CAD build for the part. Positions are in the model's coordinates, mm. A direction names the side the tool comes from. Give positions to 0.01 mm unless a question says otherwise; leave off trailing zeros. Loops run counter-clockwise (first coordinate to the right, second up) from the corner with the lowest first, then second, coordinate; pieces in that order, holes last.
```python
from build123d import *

# Parameters (mm, degrees)
F1_DEPTH = 6
F3_DEPTH = 2
F4_R     = 2.25
F5_DEPTH = 8.001
F6_R     = 3.75
F7_DEPTH = 2
F8_SIZE  = 3


with BuildPart() as f1:
    # F0 (on Top) → F1 (new body)
    with BuildSketch(Plane.XY):
        Polygon((0, 40), (0, 0), (60, 0), (60, 20), (20, 40), align=None)
    extrude(amount=F1_DEPTH)

    # F2 (on face) → F3 (join)
    with BuildSketch(Plane.XY.offset(6)):
        Polygon((12.71, 40), (7.29, 40), (7.29, 0), (10, 0), (12.71, 0), align=None)
        Polygon((60, 7.29), (60, 12.71), (20, 12.71), (20, 10), (20, 7.29), align=None)
    extrude(amount=F3_DEPTH)

    # F4 (on face) → F5 (cut, through all)
    with BuildSketch(Plane(origin=(0, 0, 0), x_dir=(1, 0, 0), z_dir=(0, 0, -1))):
        with Locations((10, -10)):
            Circle(F4_R)
        with Locations((50, -10)):
            Circle(F4_R)
        with Locations((10, -30)):
            Circle(F4_R)
        with Locations((30, -10)):
            Circle(F4_R)
    extrude(amount=-F5_DEPTH, mode=Mode.SUBTRACT)

    # F6 (on face) → F7 (cut)
    with BuildSketch(Plane(origin=(0, 0, 0), x_dir=(1, 0, 0), z_dir=(0, 0, -1))):
        with Locations((10, -10)):
            Circle(F6_R)
        with Locations((30, -10)):
            Circle(F6_R)
        with Locations((50, -10)):
            Circle(F6_R)
        with Locations((10, -30)):
            Circle(F6_R)
    extrude(amount=-F7_DEPTH, mode=Mode.SUBTRACT)

    # F8
    f8_edges = [f1.edges().sort_by_distance(p)[0] for p in [
        (30, 0, 0),
        (0, 20, 0),
        (60, 10, 0),
        (10, 40, 0),
        (40, 30, 0),
    ]]
    chamfer(f8_edges, length=F8_SIZE)


solid = f1.part
```
1. Saw through at D-D, the plane z = 4. List the corners of the cut face in (x, y).
Responses:
outline: (0, 0) - (60, 0) - (60, 20) - (20, 40) - (0, 40) - close; hole circle Ø4.5 at (10, 10); hole circle Ø4.5 at (10, 30); hole circle Ø4.5 at (30, 10); hole circle Ø4.5 at (50, 10)
2. Drop flat-ended pins along their axis: pin 1 (1 mm diameter, centred on x = 30.5, y = 11.5, fed in from -Z); pin 2 (1.6 mm diameter, centred on x = 44.5, z = 7.5, fed in from +Y); pin 3 (12 mm diameter, centred on x = 27, y = 19, fed in from +Z); pin 4 (2 mm diameter, centred on y = 18, z = 7.5, fed in from -X). Give the stop position or say it passes through.
Responses:
pin 1: passes through
pin 2: stops at y = 12.71
pin 3: stops at z = 6
pin 4: stops at x = 7.29
3. Tool access for faces 4 (the face through (7.29, 20, 7)), 5 (the face through (20, 10, 7)), 6 (the face through (40, 7.29, 7)), 7 (the face through (12, 32, 2)): list every direction of +Z, -Z, +X, -X, +Y, -Y with a clear straight run to the whole face (end or side of a thin tool).
Responses:
face 4: +Z, -X, +Y, -Y
face 5: +Z, +Y, -Y
face 6: +Z, +X, -Y
face 7: -Z
4. Saw through at C-C, the plane y = 29. List the corners of the cut face in (x, z), and give its area (3 significant figures).
Responses:
outline: (0, 3) - (3, 0) - (6.39, 0) - (6.39, 2) - (7.98, 2) - (7.98, 8) - (7.29, 8) - (7.29, 6) - (0, 6) - close; (12.02, 2) - (13.61, 2) - (13.61, 0) - (35.29, 0) - (42, 3) - (42, 6) - (12.71, 6) - (12.71, 8) - (12.02, 8) - close
area: 210 mm2
5. Saw through at B-B, the plane x = 10. List the corners of the cut face in (y, z), and give its area (3 significant figures).
Responses:
outline: (0, 3) - (3, 0) - (6.25, 0) - (6.25, 2) - (7.75, 2) - (7.75, 8) - (0, 8) - close; (12.25, 2) - (13.75, 2) - (13.75, 0) - (26.25, 0) - (26.25, 2) - (27.75, 2) - (27.75, 8) - (12.25, 8) - close; (32.25, 2) - (33.75, 2) - (33.75, 0) - (37, 0) - (40, 3) - (40, 8) - (32.25, 8) - close
area: 227 mm2
6. Probe line 1 along Y through (x, z) = (10, 5.15); line 2 along X through (y, z) = (10, 6.15); line 3 along X through (y, z) = (30, 4). List the from-to ranges inside material, lowest first.
Responses:
line 1: y = 0 to 7.75, 12.25 to 27.75, 32.25 to 40
line 2: x = 7.29 to 7.75, 12.25 to 12.71, 20 to 27.75, 32.25 to 47.75, 52.25 to 60
line 3: x = 0 to 7.75, 12.25 to 40
7. Pull direction Y, two halves, no side cores. Call faces 1 (the face through (4, 20, 6)), 2 (the face through (46.254, 9.835, 0.986)), 3 (the face through (30, 0, 4)): released by +Y, released by -Y, zero draft, split by the parting line, or undercut.
Responses:
face 1: zero draft
face 2: undercut
face 3: released by -Y
8. Saw through at A-A, the plane z = 7. List the corners of the cut face in (x, y).
Responses:
outline: (7.29, 0) - (12.71, 0) - (12.71, 40) - (7.29, 40) - close; (20, 7.29) - (60, 7.29) - (60, 12.71) - (20, 12.71) - close; hole circle Ø4.5 at (10, 10); hole circle Ø4.5 at (10, 30); hole circle Ø4.5 at (30, 10); hole circle Ø4.5 at (50, 10)
